```python
from build123d import *

# Parameters (mm, degrees)
SKETCH_1_R          = 1
EXTRUDE_1_DEPTH     = 6
SKETCH_2_R          = 1.75
CUT_EXTRUDE_1_DEPTH = 4
SKETCH_3_W          = 75.160479418
SKETCH_3_H          = 12
EXTRUDE_2_DEPTH     = 3
SKETCH_4_R          = 0.75
CUT_EXTRUDE_2_DEPTH = 3
SKETCH_5_W          = 5
SKETCH_5_H          = 12
SKETCH_5_W_2        = 30
CUT_EXTRUDE_3_DEPTH = 2
SKETCH_6_R          = 1
CUT_EXTRUDE_4_DEPTH = 120.23621269
SKETCH_6_3_R        = 1
SKETCH_6_3_R_2      = 1.75
CUT_EXTRUDE_5_DEPTH = 1


with BuildPart() as part:
    # 草图1 → 凸台-拉伸1 (new body)
    with BuildSketch(Plane.XY):
        with BuildLine():
            Line((0, -11.591109915), (26.368582626, -110))
            Line((26.368582626, -110), (32.580239709, -110))
            Line((32.580239709, -110), (2.897777479, 0.776457135))
            ThreePointArc((2.897777479, 0.776457135), (0, 3), (-2.897777479, 0.776457135))
            Line((-2.897777479, 0.776457135), (-32.580239709, -110))
            Line((-32.580239709, -110), (-26.368582626, -110))
            Line((-26.368582626, -110), (0, -11.591109915))
        make_face()
        with Locations((13.665408814, -51)):
            Circle(SKETCH_1_R, mode=Mode.SUBTRACT)
        Circle(SKETCH_1_R, mode=Mode.SUBTRACT)
        with Locations((-13.665408814, -51)):
            Circle(SKETCH_1_R, mode=Mode.SUBTRACT)
    extrude(amount=EXTRUDE_1_DEPTH)

    # 草图2 → 切除-拉伸1 (cut)
    with BuildSketch(Plane(origin=(0, 0, 0), x_dir=(-1, 0, 0), z_dir=(0, 0, -1))):
        Circle(SKETCH_2_R)
        with Locations((13.665408814, -51)):
            Circle(SKETCH_2_R)
        with Locations((-13.665408814, -51)):
            Circle(SKETCH_2_R)
    extrude(amount=-CUT_EXTRUDE_1_DEPTH, mode=Mode.SUBTRACT)

    # 草图3 → 凸台-拉伸2 (add)
    with BuildSketch(Plane.XZ.offset(110)):
        Rectangle(SKETCH_3_W, SKETCH_3_H)
    extrude(amount=EXTRUDE_2_DEPTH)

    # 草图4 → 切除-拉伸2 (cut)
    with BuildSketch(Plane.XY.offset(6)):
        with Locations((-27.59876682, -103)):
            Circle(SKETCH_4_R)
        with Locations((27.59876682, -103)):
            Circle(SKETCH_4_R)
    extrude(amount=-CUT_EXTRUDE_2_DEPTH, mode=Mode.SUBTRACT)

    # 草图5 → 切除-拉伸3 (cut)
    with BuildSketch(Plane(origin=(0, -110, 0), x_dir=(1, 0, 0), z_dir=(0, 1, 0))):
        with Locations((-35.080239709, 0)):
            Rectangle(SKETCH_5_W, SKETCH_5_H)
        with Locations((35.080239709, 0)):
            Rectangle(SKETCH_5_W, SKETCH_5_H)
        Rectangle(SKETCH_5_W_2, SKETCH_5_H)
    extrude(amount=-CUT_EXTRUDE_3_DEPTH, mode=Mode.SUBTRACT)

    # 草图6 → 切除-拉伸4 (cut, through all)
    with BuildSketch(Plane(origin=(0, -110, 0), x_dir=(1, 0, 0), z_dir=(0, 1, 0))):
        with Locations(Location((-8, 3, 0), (0, 0, 270))):
            Circle(SKETCH_6_R)
        with Locations(Location((-34.580239709, 3, 0), (0, 0, 270))):
            Circle(SKETCH_6_R)
        with Locations(Location((-18.580239709, 3, 0), (0, 0, 270))):
            Circle(SKETCH_6_R)
        with Locations(Location((8, 3, 0), (0, 0, 270))):
            Circle(SKETCH_6_R)
        with Locations(Location((18.580239709, 3, 0), (0, 0, 270))):
            Circle(SKETCH_6_R)
        with Locations(Location((34.580239709, 3, 0), (0, 0, 270))):
            Circle(SKETCH_6_R)
    extrude(amount=-CUT_EXTRUDE_4_DEPTH, mode=Mode.SUBTRACT)

    # 草图6<3> → 切除-拉伸5 (cut)
    # profile 1 of 6: a face of its own
    with BuildSketch(Plane(origin=(0, -110, 0), x_dir=(1, 0, 0), z_dir=(0, 1, 0))):
        with Locations(Location((-34.580239709, 3, 0), (0, 0, 270))):
            Circle(SKETCH_6_3_R)
    # profile 2 of 6: a face of its own
    with BuildSketch(Plane(origin=(0, -110, 0), x_dir=(1, 0, 0), z_dir=(0, 1, 0))):
        with Locations(Location((-8, 3, 0), (0, 0, 270))):
            Circle(SKETCH_6_3_R)
    # profile 3 of 6: a face of its own
    with BuildSketch(Plane(origin=(0, -110, 0), x_dir=(1, 0, 0), z_dir=(0, 1, 0))):
        with Locations(Location((8, 3, 0), (0, 0, 270))):
            Circle(SKETCH_6_3_R)
    # profile 4 of 6: a face of its own
    with BuildSketch(Plane(origin=(0, -110, 0), x_dir=(1, 0, 0), z_dir=(0, 1, 0))):
        with Locations(Location((34.580239709, 3, 0), (0, 0, 270))):
            Circle(SKETCH_6_3_R)
    # profile 5 of 6: a face of its own
    with BuildSketch(Plane(origin=(0, -110, 0), x_dir=(1, 0, 0), z_dir=(0, 1, 0))):
        with Locations(Location((18.580239709, 3, 0), (0, 0, 270))):
            Circle(SKETCH_6_3_R_2)
        with Locations(Location((18.580239709, 3, 0), (0, 0, 270))):
            Circle(SKETCH_6_3_R, mode=Mode.SUBTRACT)
    # profile 6 of 6: a face of its own
    with BuildSketch(Plane(origin=(0, -110, 0), x_dir=(1, 0, 0), z_dir=(0, 1, 0))):
        with Locations(Location((-18.580239709, 3, 0), (0, 0, 270))):
            Circle(SKETCH_6_3_R_2)
        with Locations(Location((-18.580239709, 3, 0), (0, 0, 270))):
            Circle(SKETCH_6_3_R, mode=Mode.SUBTRACT)
    extrude(amount=-CUT_EXTRUDE_5_DEPTH, mode=Mode.SUBTRACT)


solid = part.part
```
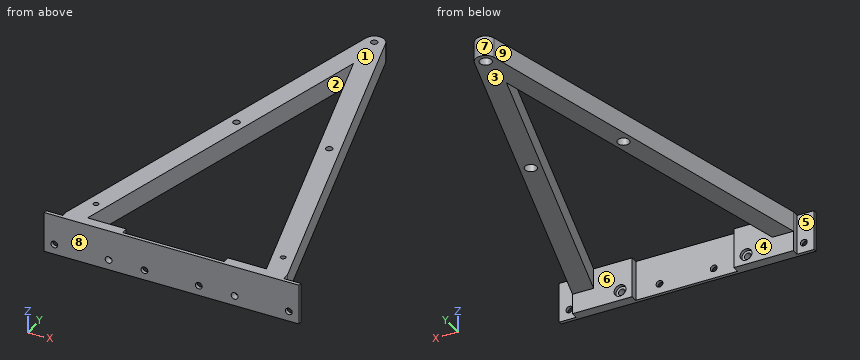
Can you work these out from the model? Positions are in its coordinate system, mm. Face numbers are marked on the shaded views. A direction names the side the tool comes from. Give positions to 0.01 mm unless a question says otherwise; leave off trailing zeros. Write each loop counter-clockwise with the first axis right and the second up, starting at its lowest first coordinate (ties: lowest second). Pieces come first, ordered by that corner, then holes. Notation, with made-up numbers: (71.5, -20) -> (125.5, -20) arc R15 cw to (125.5, -4) -> close; hole circle Ø3 at (69.25, -5). An arc over 180 degrees is marked (long way). One line per item, written item: value.
Q1. Imagine slicing it at B-B on y = -63. Please give me the cut outline in (x, z), and give its area (3 significant figures).
Results found:
outline: (-19.99, 0) -> (-13.77, 0) -> (-13.77, 6) -> (-19.99, 6) -> close; (13.77, 0) -> (19.99, 0) -> (19.99, 6) -> (13.77, 6) -> close
area: 74.5 mm^2
Q2. For P1, Ø1.6, axis at y = -111, z = 1, coming from the -X side; P2, Ø3.5, axis at x = -5, z = -2.5, coming from the +Y side; P3, Ø6, axis at x = 28, z = -3.5, coming from the +Y side, each with a flat end and sliding along its axis, tell me the tip position at first contact or that it passes through.
Results found:
P1: stops at x = -32.58
P2: stops at y = -112
P3: stops at y = -110
Q3. Imagine slicing it at A-A on z = 1.5. Please give me the cut outline in (x, y), and give its area (3 significant figures).
Results found:
outline: (-37.58, -113) -> (37.58, -113) -> (37.58, -112) -> (32.58, -112) -> (32.58, -110) -> (2.9, 0.78) arc R3 ccw to (-2.9, 0.78) -> (-32.58, -110) -> (-32.58, -112) -> (-37.58, -112) -> close; hole (-26.37, -110) -> (-15, -110) -> (-15, -112) -> (15, -112) -> (15, -110) -> (26.37, -110) -> (0, -11.59) -> close; hole circle Ø3.5 at (-13.67, -51); hole circle Ø3.5 at (0, 0); hole circle Ø3.5 at (13.67, -51)
area: 1,460 mm^2
Q4. Please list where these lines run through material, in increasing order: line 1 (X direction, y = -111.5, z = -3); line 2 (X direction, y = -103, z = 4.55); line 3 (Y direction, x = -25.5, z = -0.5). Write a range as [from, to].
Results found:
line 1: x = [-32.58, -19.58], [-17.58, -15], [15, 17.58], [19.58, 32.58]
line 2: x = [-30.7, -28.35], [-26.85, -24.49], [24.49, 26.85], [28.35, 30.7]
line 3: y = [-113, -110]
Q5. We'd pull the mould along X, two halves only. Please class the marked faces 6, 7, 8 and 9: +X half, -X half, draft (parallel to the pull), parting line (faces both ways), or undercut.
Results found:
face 6: undercut
face 7: parting line
face 8: draft
face 9: -X half
Q6. Which directions (+Z, -Z, +X, -X, +Y, -Y) give clear straight access to the entire face, cutting with the end or side of a thin tool? Please do the marked faces 1, 2, 3, 4 and 5.
Results found:
face 1: +Z, +X, -X, +Y, -Y
face 2: +Z, -Z
face 3: -Z, +X, -X, +Y
face 4: -Z
face 5: +Z, -Z, -X, +Y
